For this review, take the finished solid that the model builds, in its own axes (mm). A direction names the side the tool comes from. Give positions to 0.01 mm unless a question says otherwise; leave off trailing zeros. Write each loop counter-clockwise with the first axis right and the second up, starting at its lowest first coordinate (ties: lowest second). Pieces come first, ordered by that corner, then holes. Notation, with made-up numbers: (86.25, -23) -> (112.25, -23) arc R20 cw to (112.25, -4) -> close; hole circle Ø8 at (33.25, -23). An arc over 180 degrees is marked (long way). Write item = value, one per line.
```python
from build123d import *

# Parameters (mm, degrees)
BOSS_EXTRUDE1_DEPTH = 25
CUT_EXTRUDE1_DEPTH  = 25
SKETCH3_R           = 3
CUT_EXTRUDE2_DEPTH  = 25


with BuildPart() as part:
    # Sketch1 → Boss-Extrude1 (new body)
    with BuildSketch(Plane.XY):
        with BuildLine():
            Line((-19.099339108, 23.459186619), (-19.099339108, -11.540813381))
            ThreePointArc((-19.099339108, -11.540813381), (-18.51355267, -12.955026943), (-17.099339108, -13.540813381))
            Line((-17.099339108, -13.540813381), (17.900660892, -13.540813381))
            Line((17.900660892, -13.540813381), (17.900660892, -11.540813381))
            Line((17.900660892, -11.540813381), (-15.099339108, -11.540813381))
            ThreePointArc((-15.099339108, -11.540813381), (-16.51355267, -10.955026943), (-17.099339108, -9.540813381))
            Line((-17.099339108, -9.540813381), (-17.099339108, 23.459186619))
            Line((-17.099339108, 23.459186619), (-19.099339108, 23.459186619))
        make_face()
    extrude(amount=BOSS_EXTRUDE1_DEPTH)

    # Sketch2 → Cut-Extrude1 (cut)
    with BuildSketch(Plane.ZY.offset(19.099339108)):
        with BuildLine():
            Line((6, -1.040813381), (6, 12.959186619))
            ThreePointArc((6, 12.959186619), (12.5, 19.459186619), (19, 12.959186619))
            Line((19, 12.959186619), (19, -1.040813381))
            ThreePointArc((19, -1.040813381), (12.5, -7.540813381), (6, -1.040813381))
        make_face()
    extrude(amount=-CUT_EXTRUDE1_DEPTH, mode=Mode.SUBTRACT)

    # Sketch3 → Cut-Extrude2 (cut)
    with BuildSketch(Plane.XZ.offset(13.540813381)):
        with Locations((0.400660892, 12.5)):
            Circle(SKETCH3_R)
        with BuildLine():
            Line((5.400660892, 6), (5.400660892, 19))
            ThreePointArc((5.400660892, 19), (8.400660892, 22), (11.400660892, 19))
            Line((11.400660892, 19), (11.400660892, 6))
            ThreePointArc((11.400660892, 6), (8.400660892, 3), (5.400660892, 6))
        make_face()
        with BuildLine():
            Line((-11.002045654, 6), (-11.002045654, 19))
            ThreePointArc((-11.002045654, 19), (-8.002045654, 22), (-5.002045654, 19))
            Line((-5.002045654, 19), (-5.002045654, 6))
            ThreePointArc((-5.002045654, 6), (-8.002045654, 3), (-11.002045654, 6))
        make_face()
    extrude(amount=-CUT_EXTRUDE2_DEPTH, mode=Mode.SUBTRACT)


solid = part.part
```
(1) The part is to be moulded in two halves that separate along X. For faces 1 (the face through (-5.002, -13, 13)), 2 (the face through (-18.53, -12.94, 12.32)), 3 (the face through (-18.11, -7.54, 12.64)), say which applies: released by +X, released by -X, zero draft, split by the parting line, or undercut.
Answers below:
face_1 = undercut
face_2 = released by -X
face_3 = zero draft
(2) Take a section at D-D (z = 22.75). Write out the cut boundary in (x, y).
Answers below:
outline = (-19.1, -11.54) arc R2 ccw to (-17.1, -13.54) -> (17.9, -13.54) -> (17.9, -11.54) -> (-15.1, -11.54) arc R2 cw to (-17.1, -9.54) -> (-17.1, 23.46) -> (-19.1, 23.46) -> close
(3) Take a section at A-A (z = 12.5). Write out the cut boundary in (x, y).
Answers below:
outline = (-19.1, -11.54) arc R2 ccw to (-17.1, -13.54) -> (-11, -13.54) -> (-11, -11.54) -> (-15.1, -11.54) arc R2 cw to (-17.1, -9.54) -> (-17.1, -7.54) -> (-19.1, -7.54) -> close; (-19.1, 19.46) -> (-17.1, 19.46) -> (-17.1, 23.46) -> (-19.1, 23.46) -> close; (-5, -13.54) -> (-2.6, -13.54) -> (-2.6, -11.54) -> (-5, -11.54) -> close; (3.4, -13.54) -> (5.4, -13.54) -> (5.4, -11.54) -> (3.4, -11.54) -> close; (11.4, -13.54) -> (17.9, -13.54) -> (17.9, -11.54) -> (11.4, -11.54) -> close
(4) To check wall thickness, follow probe 1 along Y at (x, z) = (-4.5, 4); probe 2 along X at (y, z) = (20, 21). State the ranges of each line that lie inside material, in increasing order.
Answers below:
probe_1 = -13.54 to -11.54
probe_2 = -19.1 to -17.1
(5) Tool access review of faces 4 (the face through (5.401, -13, 12)), 5 (the face through (-17.099, 7, 4)), 6 (the face through (-18.113, 19.458, 12.357)): name each direction out of +Z, -Z, +X, -X, +Y, -Y from which nothing blocks a thin tool from reaching the whole face with its end or side.
Answers below:
face_4 = +Y, -Y
face_5 = +Z, -Z, +X, +Y
face_6 = +X, -X
(6) Take a section at C-C (x = -8.5). Write out the cut boundary in (y, z).
Answers below:
outline = (-13.54, 0) -> (-11.54, 0) -> (-11.54, 3.04) -> (-13.54, 3.04) -> close; (-13.54, 21.96) -> (-11.54, 21.96) -> (-11.54, 25) -> (-13.54, 25) -> close
(7) Take a section at B-B (y = 9). Write out the cut boundary in (x, z), plus the area to 3 significant figures.
Answers below:
outline = (-19.1, 0) -> (-17.1, 0) -> (-17.1, 6) -> (-19.1, 6) -> close; (-19.1, 19) -> (-17.1, 19) -> (-17.1, 25) -> (-19.1, 25) -> close
area = 24.0 mm^2
(8) For pin 1 (5 mm diameter, centred on x = 0.4, z = 12.5, fed in from -Y); pin 2 (10 mm diameter, centred on x = -10.5, z = 17.5, fed in from +Y); pin 3 (4 mm diameter, centred on y = -2, z = 21.5, fed in from +X); pin 4 (1 mm diameter, centred on y = -12.5, z = 13, fed in from -X), all flat-tipped, find the tip position at first contact; note any pin that passes through.
Answers below:
pin_1 = through
pin_2 = -11.5
pin_3 = -17.1
pin_4 = -19.05
